```python
from build123d import *

# Parameters (mm, degrees)
F0_W     = 152.4
F0_H     = 152.4
F0_W_2   = 114.3
F0_H_2   = 114.3
F1_DEPTH = 6.35
F2_D     = 3.175
F3_R     = 2.54


with BuildPart() as f1:
    # F0 (on Top) → F1 (new body)
    with BuildSketch(Plane.XY):
        Rectangle(F0_W, F0_H)
        Rectangle(F0_W_2, F0_H_2, mode=Mode.SUBTRACT)
    extrude(amount=F1_DEPTH)

    # F2 (through all)
    with Locations(Plane(origin=(0, 0, 0), x_dir=(1, 0, 0), z_dir=(0, 0, -1))):
        with Locations((-66.675, 66.675), (-38.1, 66.675), (38.1, 66.675), (66.675, 66.675), (66.675, 38.1), (66.675, -38.1), (66.675, -66.675), (38.1, -66.675), (-38.1, -66.675), (-66.675, -66.675), (-66.675, -38.1), (-66.675, 38.1)):
            Hole(F2_D / 2)

    # F3
    f3_edges = [f1.edges().sort_by_distance(p)[0] for p in [
        (-76.2, -76.2, 3.175),
        (76.2, -76.2, 3.175),
        (76.2, 76.2, 3.175),
        (-76.2, 76.2, 3.175),
    ]]
    fillet(f3_edges, radius=F3_R)


solid = f1.part
```
Geometry check sheet. Reference: the model listing, model coordinates, mm. A direction names the side the tool comes from. Give positions to 0.01 mm unless a question says otherwise; leave off trailing zeros. Order: outer loops, then holes, each group sorted by start corner. A loop starts at its lowest first (then second) coordinate and runs counter-clockwise, first axis right, second up.
1. Access from +Z, -Z, +X, -X, +Y, -Y to the whole of each face (thin tool, end or side, straight path). Record for faces 5 (the face through (-1, -76.2, 3)), 6 (the face through (-1, -57.15, 3)).
2. Thickness scan on L1, parallel to Y at x = -67, z = 2; L2, parallel to X at y = 38.1, z = 1.5; L3, parallel to X at y = 44, z = 1.25. Record the ranges inside material, lowest first.
3. Release check for a two-part mould opening along X. For faces 1 (the face through (-57.15, -1, 3)), 2 (the face through (-76.2, -1, 3)), 3 (the face through (-69, 1, 6.35)), 4 (the face through (57.15, -1, 3)) record: pulls with the +X half, pulls with the -X half, needs draft (parallel to the pull), parting line crosses it, or undercut.
4. Section check C-C, the plane z = 2.25. Give the number of separate pieces and of enclosed holes in the cut face, and give its area (3 significant figures).
5. Section check A-A, the plane y = 32.5. Enter the section's corners in (x, z), and give its area (3 significant figures).
6. Gauge pin test, flat end, axial feed: pin 1 Ø3.5 at (x, y) = (-66.675, -66.675) entering from -Z. Record the tip position at first contact, or that the pin passes through.
Values follow:
1. face 5: +Z, -Z, +X, -X, -Y
1. face 6: +Z, -Z
2. L1: y = -76.2 to -68.23, -65.12 to -39.65, -36.55 to 36.55, 39.65 to 65.12, 68.23 to 76.2
2. L2: x = -76.2 to -68.26, -65.09 to -57.15, 57.15 to 65.09, 68.26 to 76.2
2. L3: x = -76.2 to -57.15, 57.15 to 76.2
3. face 1: undercut
3. face 2: pulls with the -X half
3. face 3: needs draft
3. face 4: undercut
4. separate pieces: 1
4. enclosed holes: 13
4. area: 10,100 mm2
5. outline: (-76.2, 0) - (-57.15, 0) - (-57.15, 6.35) - (-76.2, 6.35) - close; (57.15, 0) - (76.2, 0) - (76.2, 6.35) - (57.15, 6.35) - close
5. area: 242 mm2
6. pin 1: stops at z = 0
